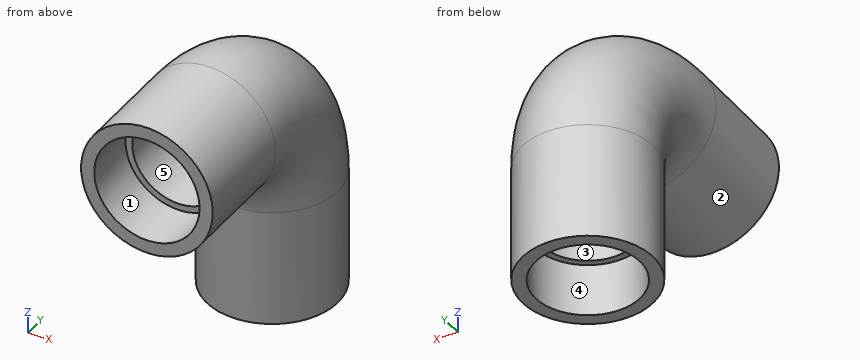
from build123d import *

# Parameters (mm, degrees)
F0_R     = 15.875
F0_R_2   = 11.1125
F3_R     = 12.7
F4_DEPTH = 12.7
F5_R     = 12.7
F6_DEPTH = 12.7


with BuildPart() as f2:
    # F2: sweep along a path in F1
    with BuildLine(Plane.YZ) as f2_path:
        Line((0, 0), (25.4, 0))
        ThreePointArc((25.4, 0), (43.3605122421, -7.4394877579), (50.8, -25.4))
        Line((50.8, -25.4), (50.8, -53.591504693))
    # F0 (on Front) → F2 (sweep)
    with BuildSketch(Plane.XZ):
        Circle(F0_R)
        Circle(F0_R_2, mode=Mode.SUBTRACT)
    sweep(path=f2_path.line)

    # F3 (on Front) → F4 (cut)
    with BuildSketch(Plane.XZ):
        Circle(F3_R)
    extrude(amount=-F4_DEPTH, mode=Mode.SUBTRACT)

    # F5 (on face) → F6 (cut)
    with BuildSketch(Plane(origin=(0, 0, -53.591504693), x_dir=(1, 0, 0), z_dir=(0, 0, -1))):
        with Locations((0, -50.8)):
            Circle(F5_R)
    extrude(amount=-F6_DEPTH, mode=Mode.SUBTRACT)


solid = f2.part
Can you work these out from the model? Positions are in its coordinate system, mm. Face numbers are marked on the shaded views. A direction names the side the tool comes from. Give positions to 0.01 mm unless a question says otherwise; leave off trailing zeros. Loops run counter-clockwise (first coordinate to the right, second up) from the corner with the lowest first, then second, coordinate; pieces in that order, holes last. Notation, with made-up numbers: (-8.5, 75) - (25.5, 75) arc R32 cw to (25.5, 103) - close; hole circle Ø3 at (82.25, 7). An arc over 180 degrees is marked (long way). Return JSON: item names as keys, results as strings.
1. I'm going to push flat-ended pins straight in: pin 1 Ø6 at (x, z) = (12.5, -18) entering from -Y; pin 2 Ø2 at (x, y) = (-4.5, 12.5) entering from +Z; pin 3 Ø5 at (y, z) = (51, -9.5) entering from -X. Where does each tip first touch, or does it pass through?
Output values:
{"pin 1": "stops at y = 34.79", "pin 2": "stops at z = 15.48", "pin 3": "stops at x = -15.72"}
2. I want a section at A-A on x = -7.5. Please give me the cut outline in (y, z).
Output values:
{"outline": "(0, -13.99) - (25.4, -13.99) arc R11.41 cw to (36.81, -25.4) - (36.81, -53.59) - (40.55, -53.59) - (40.55, -40.89) - (42.6, -40.89) - (42.6, -25.4) arc R17.2 ccw to (25.4, -8.2) - (12.7, -8.2) - (12.7, -10.25) - (0, -10.25) - close; (0, 10.25) - (12.7, 10.25) - (12.7, 8.2) - (25.4, 8.2) arc R33.6 cw to (59, -25.4) - (59, -40.89) - (61.05, -40.89) - (61.05, -53.59) - (64.79, -53.59) - (64.79, -25.4) arc R39.39 ccw to (25.4, 13.99) - (0, 13.99) - close"}
3. I want a section at C-C on y = 10.5. Please give me the cut outline in (x, z) (3 decimals).
Output values:
{"outline": "circle Ø31.75 at (0, 0); hole circle Ø25.4 at (0, 0)"}
4. We'd pull the mould along X, two halves only. Please class the marked faces 1, 2 and 3: +X half, -X half, draft (parallel to the pull), parting line (faces both ways), or undercut.
Output values:
{"face 1": "undercut", "face 2": "parting line", "face 3": "undercut"}
5. If I drill on line 1 (Z direction, x = 0, y = 3.5) (3 decimals); line 2 (Z direction, x = 0, y = 18) (1 decimal), over which ranges is the centre line in solid material (lowest first)?
Output values:
{"line 1": "z = -15.875 to -12.7, 12.7 to 15.875", "line 2": "z = -15.9 to -11.1, 11.1 to 15.9"}
6. For the marked faces 4 and 5, which set-ups out of +Z, -Z, +X, -X, +Y, -Y let a thin tool reach every point of the face, with its end or its side?
Output values:
{"face 4": "-Z", "face 5": "-Y"}
7. I want a section at B-B on z = -44.5. Please give me the cut outline in (x, y) (3 decimals), and give its area (3 significant figures).
Output values:
{"outline": "circle Ø31.75 at (0, 50.8); hole circle Ø25.4 at (0, 50.8)", "area": "285 mm²"}
